Here's how the part is built. I have some questions about the finished solid (model axes, mm). A direction names the side the tool comes from. Give positions to 0.01 mm unless a question says otherwise; leave off trailing zeros. Write each loop counter-clockwise with the first axis right and the second up, starting at its lowest first coordinate (ties: lowest second). Pieces come first, ordered by that corner, then holes. Notation, with made-up numbers: (82.25, 37) - (96.25, 37) arc R24 cw to (96.25, 72) - close; hole circle Ø8 at (-13, 80.25). An arc over 180 degrees is marked (long way). Use a Markdown table: item, result.
```python
from build123d import *

# Parameters (mm, degrees)
F0_R     = 1.6
F2_DEPTH = 1.6764
F1_W     = 15.75
F1_H     = 11.94
F3_DEPTH = 11.2776
F1_W_2   = 13.46
F1_H_2   = 9.02
F4_DEPTH = 10.6172
F5_R     = 4.3815
F1_W_3   = 20.8788
F1_H_3   = 2.54
F1_W_4   = 15.748
F1_W_5   = 25.908
F1_W_6   = 20.828
F6_DEPTH = 8.3566


with BuildPart() as f2:
    # F0 (on Top) → F2 (new body)
    with BuildSketch(Plane.XY):
        Polygon((30.23, 26.67), (-34.29, 26.67), (-34.29, -26.67), (31.75, -26.67), (31.75, -24.13), (34.29, -21.59), (34.29, 11.18), (31.75, 13.72), (31.75, 25.15), align=None)
        with Locations((-20.32, -24.13)):
            Circle(F0_R, mode=Mode.SUBTRACT)
        with Locations((31.75, -19.05)):
            Circle(F0_R, mode=Mode.SUBTRACT)
        with Locations((-19.05, 24.13)):
            Circle(F0_R, mode=Mode.SUBTRACT)
        with Locations((31.75, 8.89)):
            Circle(F0_R, mode=Mode.SUBTRACT)
    extrude(amount=-F2_DEPTH)

    # F1 (on Top) → F3 (join)
    with BuildSketch(Plane.XY):
        with Locations((-32.765, 11.43)):
            Rectangle(F1_W, F1_H)
    extrude(amount=F3_DEPTH)

    # F1 (on Top) → F4 (join)
    with BuildSketch(Plane.XY):
        with Locations((-29.34, -18.86)):
            Rectangle(F1_W_2, F1_H_2)
    extrude(amount=F4_DEPTH)

    # F5
    f5_edges = [f2.edges().sort_by_distance(p)[0] for p in [
        (-29.34, -23.37, 10.6172),
        (-29.34, -14.35, 10.6172),
    ]]
    fillet(f5_edges, radius=F5_R)

    # F1 (on Top) → F6 (join)
    with BuildSketch(Plane.XY):
        with Locations((2.2606, -24.13)):
            Rectangle(F1_W_3, F1_H_3)
        with Locations((23.0124, -24.13)):
            Rectangle(F1_W_4, F1_H_3)
        with Locations((-3.7846, 24.13)):
            Rectangle(F1_W_5, F1_H_3)
        with Locations((20.2438, 24.13)):
            Rectangle(F1_W_6, F1_H_3)
    extrude(amount=F6_DEPTH)


solid = f2.part
```
Item 1: If we section it at A-A, the plane y = 24.13: Write out the boundary of the cut face in (x, z).
Values:
| item | result |
|---|---|
| outline | (-34.29, -1.68) - (-20.65, -1.68) - (-20.65, 0) - (-34.29, 0) - close; (-17.45, -1.68) - (31.75, -1.68) - (31.75, 0) - (30.66, 0) - (30.66, 8.36) - (9.83, 8.36) - (9.83, 0) - (9.17, 0) - (9.17, 8.36) - (-16.74, 8.36) - (-16.74, 0) - (-17.45, 0) - close |
Item 2: If we section it at C-C, the plane x = 16: Write out the boundary of the cut face in (y, z), plus the area to 3 significant figures.
Values:
| item | result |
|---|---|
| outline | (-26.67, -1.68) - (26.67, -1.68) - (26.67, 0) - (25.4, 0) - (25.4, 8.36) - (22.86, 8.36) - (22.86, 0) - (-22.86, 0) - (-22.86, 8.36) - (-25.4, 8.36) - (-25.4, 0) - (-26.67, 0) - close |
| area | 132 mm2 |
Item 3: I need wall thicknesses on line 1 along Y through (x, z) = (8, 4.5); line 2 along Y through (x, z) = (-19.05, -0.85); line 3 along Y through (x, z) = (-20.32, -1.05). Which ranges of each line are inside material? Lowest first, please. Write a range as [from, to].
Values:
| item | result |
|---|---|
| line 1 | y = [-25.4, -22.86], [22.86, 25.4] |
| line 2 | y = [-26.67, -25.1], [-23.16, 22.53], [25.73, 26.67] |
| line 3 | y = [-26.67, -25.73], [-22.53, 23.16], [25.1, 26.67] |
Item 4: Will these pins go through, and if not, where does the flat tip stop? pin 1 Ø1.8 at (y, z) = (-25, -1) entering from +X; pin 2 Ø3 at (x, y) = (3.5, -23.5) entering from +Z; pin 3 Ø2 at (y, z) = (-23.5, 3) entering from -X; pin 4 Ø4 at (x, y) = (-19.05, 24.13) entering from -Z.
Values:
| item | result |
|---|---|
| pin 1 | stops at x = 31.78 |
| pin 2 | stops at z = 8.36 |
| pin 3 | stops at x = -36.07 |
| pin 4 | stops at z = -1.68 |
Item 5: If we section it at D-D, the plane y = 8.89: Write out the boundary of the cut face in (x, z), plus the area to 3 significant figures.
Values:
| item | result |
|---|---|
| outline | (-40.64, 0) - (-34.29, 0) - (-34.29, -1.68) - (30.15, -1.68) - (30.15, 0) - (-24.89, 0) - (-24.89, 11.28) - (-40.64, 11.28) - close; (33.35, -1.68) - (34.29, -1.68) - (34.29, 0) - (33.35, 0) - close |
| area | 287 mm2 |
Item 6: Thinking about a two-plate mould opening in Y: for faces 5 (the flat face through (23, -25.4, 4)), 6 (the flat face through (-29, -14.35, 3)), 7 (the flat face through (-22.61, -19, 5)), which applies, +Y half, -Y half, draft (parallel to the pull), parting line (faces both ways), or undercut?
Values:
| item | result |
|---|---|
| face 5 | -Y half |
| face 6 | undercut |
| face 7 | draft |
Item 7: If we section it at B-B, the plane z = 1.5: Write out the boundary of the cut face in (x, y), plus the area to 3 significant figures.
Values:
| item | result |
|---|---|
| outline | (-40.64, 5.46) - (-24.89, 5.46) - (-24.89, 17.4) - (-40.64, 17.4) - close; (-36.07, -23.37) - (-22.61, -23.37) - (-22.61, -14.35) - (-36.07, -14.35) - close; (-16.74, 22.86) - (9.17, 22.86) - (9.17, 25.4) - (-16.74, 25.4) - close; (-8.18, -25.4) - (12.7, -25.4) - (12.7, -22.86) - (-8.18, -22.86) - close; (9.83, 22.86) - (30.66, 22.86) - (30.66, 25.4) - (9.83, 25.4) - close; (15.14, -25.4) - (30.89, -25.4) - (30.89, -22.86) - (15.14, -22.86) - close |
| area | 521 mm2 |
Item 8: For faces 1 (the flat face through (30.658, 24, 4)), 2 (the flat face through (-4, 25.4, 4)), 3 (the flat face through (-29, -23.37, 3)), 4 (the flat face through (2, -22.86, 4)), which set-ups out of +Z, -Z, +X, -X, +Y, -Y let a thin tool reach every point of the face, with its end or its side?
Values:
| item | result |
|---|---|
| face 1 | +Z, +X, +Y |
| face 2 | +Z, +X, -X, +Y |
| face 3 | +Z, -X, -Y |
| face 4 | +Z, +X |
